Here's the drawing with two shaded views (mm, measured from the low corner). I have some questions. A direction names the side the tool comes from. Coordinates: 2 decimals unless noted, no trailing zeros. Loops run counter-clockwise (first coordinate to the right, second up) from the corner with the lowest first, then second, coordinate; pieces in that order, holes last. Notation, with made-up numbers: (-19.5, 30) - (30.5, 30) arc R20 ccw to (30.5, 44) - close; hole circle Ø10 at (-6.75, 67.5). An arc over 180 degrees is marked (long way). One line per item, written item: value. Start each with the question number.
(1) If we section it at B-B on z = 13: Write out the boundary of the cut face in (x, y), then the cut area to 3 significant figures.
(2) If we section it at A-A on y = 16.5: Write out the boundary of the cut face in (x, z) (1 decimal), then the cut area to 3 significant figures.
(3) I'm going to push flat-ended pins straight in: P1, Ø13, axis at y = 19, z = 11.5, coming from the +X side; P2, Ø3, axis at y = 21, z = 33.5, coming from the +X side (3 decimals); P3, Ø1, axis at y = 31, z = 23, coming from the -X side. Where does each tip first touch, or does it pass through?
(4) On a 3-axis mill with a long thin cutter (end or side, diameter ignored), from which of +Z, -Z, +X, -X, +Y, -Y can I reach the whole of each face in a straight line? I mean the marked faces 1, 2 and 3. Say none if no direction works.
(5) If I drill on line 1 along Z through (x, y) = (55, 25) (1 decimal); line 2 along X through (y, z) = (37.5, 28.5) (1 decimal); line 3 along X through (y, z) = (42, 22.5), over which ranges is the centre line in solid material (lowest first)? Write a range as from..to.
(6) If we section it at C-C on x = 56.5: Write out the boundary of the cut face in (y, z) (1 decimal), then the cut area to 3 significant figures.
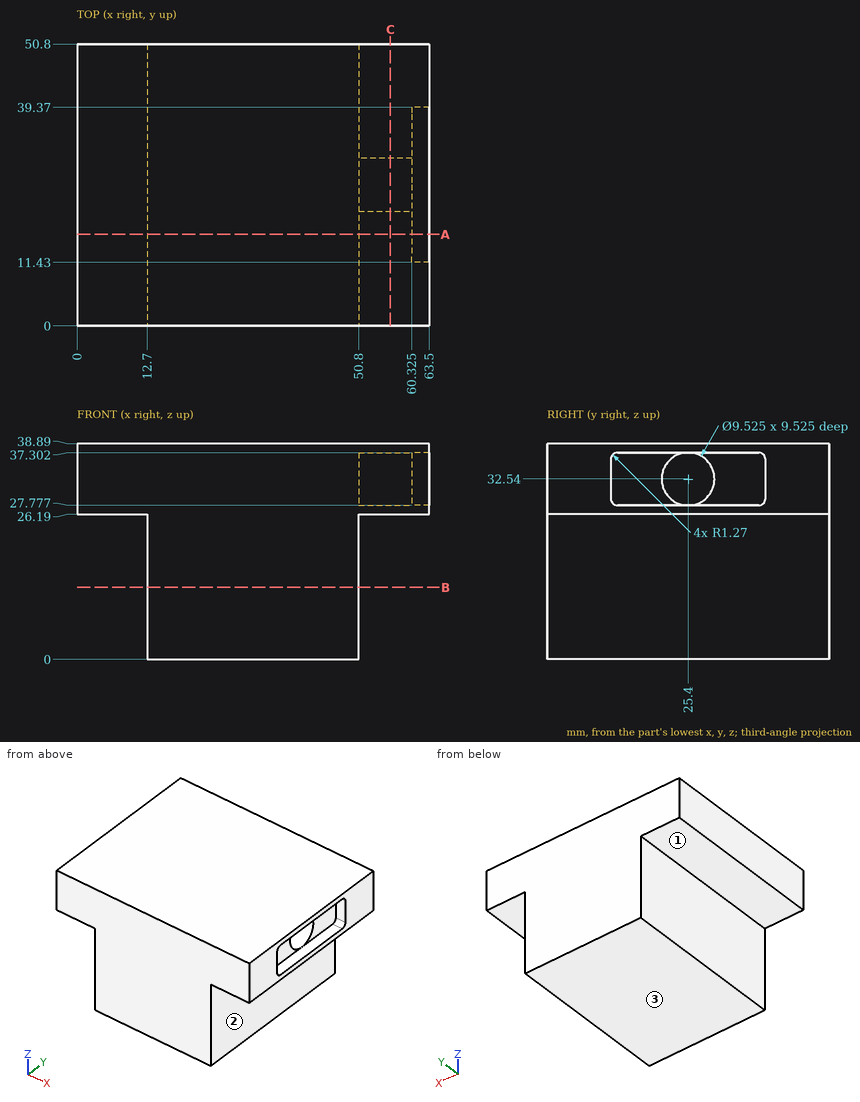
Values:
1. outline: (12.7, 0) - (50.8, 0) - (50.8, 50.8) - (12.7, 50.8) - close
1. area: 1,940 mm2
2. outline: (0, 26.2) - (12.7, 26.2) - (12.7, 0) - (50.8, 0) - (50.8, 26.2) - (63.5, 26.2) - (63.5, 27.8) - (60.3, 27.8) - (60.3, 37.3) - (63.5, 37.3) - (63.5, 38.9) - (0, 38.9) - close
2. area: 1,770 mm2
3. P1: stops at x = 50.8
3. P2: stops at x = 60.325
3. P3: stops at x = 12.7
4. face 1: -Z, -X, +Y, -Y
4. face 2: -Z, +X, +Y, -Y
4. face 3: -Z, +X, -X, +Y, -Y
5. line 1: z = 26.2..27.8, 37.3..38.9
5. line 2: x = 0..60.3
5. line 3: x = 12.7..50.8
6. outline: (0, 26.2) - (50.8, 26.2) - (50.8, 38.9) - (0, 38.9) - close; hole circle Ø9.5 at (25.4, 32.5)
6. area: 574 mm2
